```python
from build123d import *

# Parameters (mm, degrees)
SKETCH1_R           = 3.7592
SKETCH1_W           = 1.5875
SKETCH1_H           = 1.3208
BOSS_EXTRUDE1_DEPTH = 1.5875


with BuildPart() as part:
    # Sketch1 → Boss-Extrude1 (new body)
    # profile 1 of 6: a face of its own
    with BuildSketch(Plane.XY):
        with BuildLine():
            ThreePointArc((2.54, 21.59), (-3.139612663, 20.249225326), (-7.62, 16.51))
            ThreePointArc((-7.62, 16.51), (-9.508277885, 12.906092628), (-10.16, 8.89))
            Line((-10.16, 8.89), (-10.16, 4.318))
            Line((-10.16, 4.318), (-10.16, -0.889))
            Line((-10.16, -0.889), (-10.16, -2.2098))
            Line((-10.16, -2.2098), (-10.16, -3.81))
            Line((-10.16, -3.81), (9.525, -3.81))
            Line((9.525, -3.81), (9.525, -2.032))
            Line((9.525, -2.032), (8.001, -2.032))
            Line((8.001, -2.032), (8.001, 1.016))
            Line((8.001, 1.016), (9.525, 1.016))
            Line((9.525, 1.016), (9.525, 2.54))
            Line((9.525, 2.54), (9.525, 3.8608))
            Line((9.525, 3.8608), (9.525, 16.51))
            Line((9.525, 16.51), (9.525, 17.8308))
            Line((9.525, 17.8308), (9.525, 21.59))
            Line((9.525, 21.59), (2.54, 21.59))
        make_face()
        Circle(SKETCH1_R, mode=Mode.SUBTRACT)
    # profile 2 of 6: a face of its own
    with BuildSketch(Plane.XY):
        with Locations((-10.95375, -1.5494)):
            Rectangle(SKETCH1_W, SKETCH1_H)
    # profile 3 of 6: a face of its own
    with BuildSketch(Plane.XY):
        with Locations((10.31875, 17.1704)):
            Rectangle(SKETCH1_W, SKETCH1_H)
    # profile 4 of 6: a face of its own
    with BuildSketch(Plane.XY):
        with Locations((10.31875, 3.2004)):
            Rectangle(SKETCH1_W, SKETCH1_H)
    # profile 5 of 6: a face of its own
    with BuildSketch(Plane.XY):
        with BuildLine():
            ThreePointArc((-10.16, 8.89), (-9.508277885, 12.906092628), (-7.62, 16.51))
            Line((-7.62, 16.51), (-22.084921519, 16.51))
            Line((-22.084921519, 16.51), (-22.084921519, 13.081))
            Line((-22.084921519, 13.081), (-22.084921519, 4.699))
            Line((-22.084921519, 4.699), (-22.084921519, 2.212007412))
            Line((-22.084921519, 2.212007412), (-10.16, 4.318))
            Line((-10.16, 4.318), (-10.16, 8.89))
        make_face()
    # profile 6 of 6: a face of its own
    with BuildSketch(Plane.XY):
        with BuildLine():
            ThreePointArc((-10.16, 8.89), (-9.508277885, 12.906092628), (-7.62, 16.51))
            Line((-7.62, 16.51), (-22.084921519, 16.51))
            Line((-22.084921519, 16.51), (-22.084921519, 13.081))
            Line((-22.084921519, 13.081), (-22.084921519, 4.699))
            Line((-22.084921519, 4.699), (-22.084921519, 2.212007412))
            Line((-22.084921519, 2.212007412), (-10.16, 4.318))
            Line((-10.16, 4.318), (-10.16, 8.89))
        make_face()
    extrude(amount=BOSS_EXTRUDE1_DEPTH)


solid = part.part
```
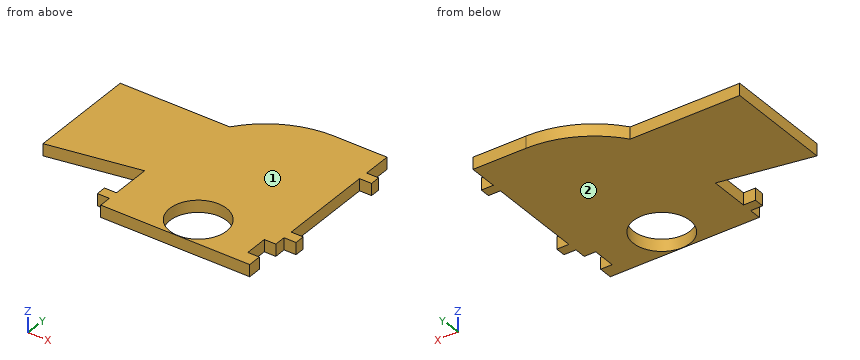
Work out the finished part from the listing and answer in its coordinate system (mm). Face numbers are marked on the shaded views. Give positions to 0.01 mm unless a question says otherwise; leave off trailing zeros. Loops run counter-clockwise (first coordinate to the right, second up) from the corner with the lowest first, then second, coordinate; pieces in that order, holes last. Notation, with made-up numbers: (-7, -29.75) -> (-2, -29.75) arc R31 ccw to (-2, 1.25) -> close; hole circle Ø11 at (39.25, 5). An arc over 180 degrees is marked (long way). Use CSV: the item, a comma, the result in double quotes.
1. The mould has two halves that part along Z. Classify the marked faces 1 and 2: +Z half, -Z half, draft (parallel to the pull), parting line (faces both ways), or undercut.
Found:
face 1,"+Z half"
face 2,"-Z half"
2. The part is cut by section A-A (z = 1.3). Write down the section's boundary in (x, y) (1 decimal), then the cut area to 3 significant figures.
Found:
outline,"(-22.1, 2.2) -> (-10.2, 4.3) -> (-10.2, -0.9) -> (-11.7, -0.9) -> (-11.7, -2.2) -> (-10.2, -2.2) -> (-10.2, -3.8) -> (9.5, -3.8) -> (9.5, -2) -> (8, -2) -> (8, 1) -> (9.5, 1) -> (9.5, 2.5) -> (11.1, 2.5) -> (11.1, 3.9) -> (9.5, 3.9) -> (9.5, 16.5) -> (11.1, 16.5) -> (11.1, 17.8) -> (9.5, 17.8) -> (9.5, 21.6) -> (2.5, 21.6) arc R12.7 ccw to (-7.6, 16.5) -> (-22.1, 16.5) -> close; hole circle Ø7.5 at (0, 0)"
area,"587 mm^2"
3. Flat-ended cylindrical pins translate along their axes: pin 1 Ø0.5 at (x, z) = (-11.5, 1) entering from +Y; pin 2 Ø0.5 at (x, z) = (10.5, 1) entering from -Y; pin 3 Ø0.8 at (x, z) = (10.5, 1) entering from +Y. Find the tip coordinate at first contact, or state that the pin passes through.
Found:
pin 1,"y = 16.51"
pin 2,"y = 2.54"
pin 3,"y = 17.83"
4. The part is cut by section C-C (y = 0). Write down the section's boundary in (x, z).
Found:
outline,"(-10.16, 0) -> (-3.76, 0) -> (-3.76, 1.59) -> (-10.16, 1.59) -> close; (3.76, 0) -> (8, 0) -> (8, 1.59) -> (3.76, 1.59) -> close"
5. The part is cut by section B-B (x = -0.5). Write down the section's boundary in (y, z), then the cut area to 3 significant figures.
Found:
outline,"(-3.81, 0) -> (-3.73, 0) -> (-3.73, 1.59) -> (-3.81, 1.59) -> close; (3.73, 0) -> (21.22, 0) -> (21.22, 1.59) -> (3.73, 1.59) -> close"
area,"27.9 mm^2"
6. Straight lines are drawn through the part: line 1 (X direction, y = 0.25, z = 1.2); line 2 (Y direction, x = 9, z = 1.25); line 3 (X direction, y = 8, z = 1.2) (3 decimals). For each, find the intervals that lie inside material, in ascending order.
Found:
line 1,"-10.16 to -3.75, 3.75 to 8"
line 2,"-3.81 to -2.03, 1.02 to 21.59"
line 3,"-22.085 to 9.525"
7. The part is cut by section D-D (y = 3). Write down the section's boundary in (x, z).
Found:
outline,"(-22.08, 0) -> (-17.62, 0) -> (-17.62, 1.59) -> (-22.08, 1.59) -> close; (-10.16, 0) -> (-2.27, 0) -> (-2.27, 1.59) -> (-10.16, 1.59) -> close; (2.27, 0) -> (11.11, 0) -> (11.11, 1.59) -> (2.27, 1.59) -> close"
